Autodesk Inventor part; units mm, degrees
ref_plane "YZ Plane" through (0, 0, 0) normal (1, 0, 0) x (0, 1, 0)
ref_plane "XZ Plane" through (0, 0, 0) normal (0, 1, 0) x (-1, 0, 0)
ref_plane "XY Plane" through (0, 0, 0) normal (0, 0, 1) x (1, 0, 0)
sketch "Sketch9" plane through (0, 0, 0) normal (0, 1, 0) x (-1, 0, 0)
  line L0 (17.5, 17.5) -> (-17.5, 17.5)
  line L1 (-17.5, 17.5) -> (-17.5, -17.5)
  line L2 (-17.5, -17.5) -> (17.5, -17.5)
  line L3 (17.5, -17.5) -> (17.5, 17.5)
  line L4 (17.5, 17.5) -> (-17.5, -17.5) construction
  line L5 (-17.5, 17.5) -> (17.5, -17.5) construction
  line L6 (-15.5, 15.5) -> (15.5, 15.5)
  line L7 (15.5, 15.5) -> (15.5, -15.5)
  line L8 (15.5, -15.5) -> (-15.5, -15.5)
  line L9 (-15.5, -15.5) -> (-15.5, 15.5)
  point P0 (0, 0)
  dimension "d172" = 35
  dimension "d173" = 35
  dimension "d174" = 2
extrude "Extrusion3" add sketch "Sketch9" against normal blind 500
sketch "Sketch10" plane through (0, 0, 0) normal (1, 0, 0) x (0, 1, 0)
  line L0 (0, 17.5) -> (0, -17.5) construction
  line L1 (0, 17.5) -> (-500, 17.5) construction
  line L2 (-500, -17.5) -> (-500, 17.5) construction
  line L3 (0, -17.5) -> (-500, -17.5) construction
  line L4 (-483, 8.5) -> (-466, 8.5)
  line L5 (-466, 8.5) -> (-466, -8.5)
  line L6 (-466, -8.5) -> (-483, -8.5)
  line L7 (-483, -8.5) -> (-483, 8.5)
  line L8 (-483, 8.5) -> (-466, -8.5) construction
  line L9 (-466, 8.5) -> (-483, -8.5) construction
  circle A0 centre (-474.5, 0) radius 8.5
  line L10 (0, 17.5) -> (0, -17.5)
  point P0 (0, 0)
  point P1 (0, 0)
  point P2 (-500, 0)
  dimension "d177" = 17
  dimension "d178" = 17
  dimension "d191" = 17
extrude "Extrusion4" cut sketch "Sketch10" along normal through all contours A0
pattern_linear "Rectangular Pattern4" count 4 spacing 145 along (0, 1, 0) of "Extrusion4"
properties part number "ANP 1435 FDS WAY tube5" material "Stainless Steel"
Design review of the part built by this model. Coordinates are the model's own, in mm. A direction names the side the tool comes from. Give positions to 0.01 mm unless a question says otherwise; leave off trailing zeros. Write each loop counter-clockwise with the first axis right and the second up, starting at its lowest first coordinate (ties: lowest second). Pieces come first, ordered by that corner, then holes. Notation, with made-up numbers: (28.25, 25.5) -> (40.25, 25.5) arc R25 cw to (40.25, 52.5) -> close; hole circle Ø7 at (85.25, 43.5). An arc over 180 degrees is marked (long way). Answer in a Markdown table with one row per item.
(1) Consider section A-A (y = -394.5). State the section outline as (x, z) points.
Results:
| item | result |
|---|---|
| outline | (-17.5, -17.5) -> (17.5, -17.5) -> (17.5, 17.5) -> (-17.5, 17.5) -> close; hole (-15.5, -15.5) -> (15.5, -15.5) -> (15.5, 15.5) -> (-15.5, 15.5) -> close |
(2) Mouldability with a two-part tool opening along X and no side actions: class faces 4 (the flat face through (17.5, -246, 0)), 5 (the flat face through (0, -246, 15.5)), 6 (the flat face through (0, -246, -15.5)), 7 (the cylindrical face through (16, -483, 0)) as +X half, -X half, draft (parallel to the pull), parting line (faces both ways), or undercut.
Results:
| item | result |
|---|---|
| face 4 | +X half |
| face 5 | undercut |
| face 6 | undercut |
| face 7 | draft |
(3) For faces 1 (the flat face through (-15.5, -246, 0)), 2 (the cylindrical face through (16, -338, 0)), 3 (the flat face through (0, -246, -17.5)), list the 3-axis set-ups (+Z, -Z, +X, -X, +Y, -Y) from which the entire face can be reached by the end or side of a thin tool; tool diameter is ignored.
Results:
| item | result |
|---|---|
| face 1 | +Y, -Y |
| face 2 | +X |
| face 3 | -Z, +X, -X, +Y, -Y |
(4) Consider section C-C (x = -9). State the section outline as (y, z) points, then the cut area to 3 significant figures.
Results:
| item | result |
|---|---|
| outline | (-500, -17.5) -> (0, -17.5) -> (0, -15.5) -> (-500, -15.5) -> close; (-500, 15.5) -> (0, 15.5) -> (0, 17.5) -> (-500, 17.5) -> close |
| area | 2,000 mm2 |
(5) To check wall thickness, follow probe 1 along Y at (x, z) = (16, 0); probe 2 along Z at (x, y) = (8.5, -197). State the ranges of each line that lie inside material, in increasing order.
Results:
| item | result |
|---|---|
| probe 1 | -500 to -483, -466 to -338, -321 to -193, -176 to -48, -31 to 0 |
| probe 2 | -17.5 to -15.5, 15.5 to 17.5 |
(6) Clearance check with a flat-ended pin moving along its axis: pin 1 (8 mm diameter, centred on x = -0.5, z = 12.5, fed in from -Y). State where the tip first meets the part, or that it passes through.
Results:
| item | result |
|---|---|
| pin 1 | y = -500 |
(7) Consider section D-D (y = -329.5). State the section outline as (x, z) points.
Results:
| item | result |
|---|---|
| outline | (-17.5, -17.5) -> (17.5, -17.5) -> (17.5, -8.5) -> (15.5, -8.5) -> (15.5, -15.5) -> (-15.5, -15.5) -> (-15.5, 15.5) -> (15.5, 15.5) -> (15.5, 8.5) -> (17.5, 8.5) -> (17.5, 17.5) -> (-17.5, 17.5) -> close |
(8) Consider section B-B (z = 0). State the section outline as (x, y) points, then the cut area to 3 significant figures.
Results:
| item | result |
|---|---|
| outline | (-17.5, -500) -> (-15.5, -500) -> (-15.5, 0) -> (-17.5, 0) -> close; (15.5, -500) -> (17.5, -500) -> (17.5, -483) -> (15.5, -483) -> close; (15.5, -466) -> (17.5, -466) -> (17.5, -338) -> (15.5, -338) -> close; (15.5, -321) -> (17.5, -321) -> (17.5, -193) -> (15.5, -193) -> close; (15.5, -176) -> (17.5, -176) -> (17.5, -48) -> (15.5, -48) -> close; (15.5, -31) -> (17.5, -31) -> (17.5, 0) -> (15.5, 0) -> close |
| area | 1,860 mm2 |
